For this review, take the finished solid that the model builds, in its own axes (mm). A direction names the side the tool comes from. Coordinates: 2 decimals unless noted, no trailing zeros. Loops run counter-clockwise (first coordinate to the right, second up) from the corner with the lowest first, then second, coordinate; pieces in that order, holes last. Notation, with made-up numbers: (40, 81.5) - (95, 81.5) arc R31 cw to (95, 110.5) - close; hole circle Ø5 at (51, 43). An arc over 180 degrees is marked (long way). One line per item, written item: value. Start each with the question number.
1. Insertion check: pin 1 (6.5 mm diameter, centred on y = 80, z = 108.5, fed in from +X); pin 2 (10 mm diameter, centred on x = 146, y = 134, fed in from +Z); pin 3 (4 mm diameter, centred on y = 122, z = 141.5, fed in from +X); pin 4 (2.5 mm diameter, centred on y = 58, z = 110, fed in from -X). Each pin has a flat end and moves straight along its axis. Give the tip position at first contact, or say it passes through.
2. Take a section at D-D, the plane x = 80.5. State the section outline as (y, z) points.
3. Take a section at C-C, the plane z = 69.5. State the section outline as (x, y) points, and give its area (3 significant figures).
4. Take a section at A-A, the plane x = 139. State the section outline as (y, z) points, and give its area (3 significant figures).
5. The part is to be moulded in two halves that separate along Z. For faces 1 (the face through (59.972, 143.384, 82.338)), 2 (the face through (54, 99, 225)), 3 (the face through (62, 122.3, 83.7)), say which applies: released by +Z, released by -Z, zero draft, split by the parting line, or undercut.
6. Take a section at B-B, the plane x = 104.5. State the section outline as (y, z) points.
7. For faces 4 (the face through (83, 142, 37)), 5 (the face through (59.972, 109.884, 97.338)), 6 (the face through (62, 59.3, 108.7)), 7 (the face through (142, 99.75, 37)), 8 (the face through (83, 57, 37)), list the 3-axis set-ups (+Z, -Z, +X, -X, +Y, -Y) from which the entire face can be reached by the end or side of a thin tool; tool diameter is ignored.
8. To check wall thickness, follow line 1 (Y direction, x = 104.5, z = 42); line 2 (Y direction, x = 53.5, z = 110); line 3 (Z direction, x = 57, y = 121). State the ranges of each line that lie inside material, in increasing order. Write a range as from..to.
```python
from build123d import *

# Parameters (mm, degrees)
F3_DEPTH = 230
F2_W     = 108
F2_H     = 30
F2_W_2   = 100
F2_H_2   = 180
F4_DEPTH = 310
F6_START = 35
F5_R     = 1.5
F6_DEPTH = 36
F7_START = 58
F5_R_2   = 3
F7_DEPTH = 4
F8_START = -44
F2_R     = 2.5
F8_DEPTH = 98


with BuildPart() as f3:
    # F1 (on Top) → F3 (new body)
    with BuildSketch(Plane.XY):
        with BuildLine():
            Line((83, 150), (50, 150))
            Line((50, 150), (50, 50))
            Line((50, 50), (83, 50))
            Line((83, 50), (83, 65))
            Line((83, 65), (158, 65))
            Line((158, 65), (158, 99.75))
            Line((158, 99.75), (126, 99.75))
            Line((126, 99.75), (125.9985464625, 99.75))
            ThreePointArc((125.9985464625, 99.75), (83, 100), (125.9985464625, 100.25))
            Line((125.9985464625, 100.25), (126, 100.25))
            Line((126, 100.25), (158, 100.25))
            Line((158, 100.25), (158, 135))
            Line((158, 135), (83, 135))
            Line((83, 135), (83, 150))
        make_face()
    extrude(amount=F3_DEPTH)

    # F2 (on Front) → F4 (cut)
    with BuildSketch(Plane.XZ):
        with Locations((104, 15)):
            Rectangle(F2_W, F2_H)
        with Locations((108, 135)):
            Rectangle(F2_W_2, F2_H_2)
        Polygon((50, 295), (50, 225), (58, 225), (158, 225), (158, 295), align=None)
    extrude(amount=-F4_DEPTH, mode=Mode.SUBTRACT)

    # F5 (on Right) → F6 (cut)
    with BuildSketch(Plane.YZ.offset(F6_START)):
        with Locations((142, 85)):
            Circle(F5_R)
        with Locations((142, 110)):
            Circle(F5_R)
        with Locations((121, 110)):
            Circle(F5_R)
        with Locations((108.5, 100)):
            Circle(F5_R)
        with Locations((121, 85)):
            Circle(F5_R)
        with Locations((90, 100)):
            Circle(F5_R)
        with Locations((79, 85)):
            Circle(F5_R)
        with Locations((58, 110)):
            Circle(F5_R)
        with Locations((79, 110)):
            Circle(F5_R)
        with Locations((58, 85)):
            Circle(F5_R)
    extrude(amount=F6_DEPTH, mode=Mode.SUBTRACT)

    # F5 (on Right) → F7 (join)
    with BuildSketch(Plane.YZ.offset(F7_START)):
        with Locations((58, 110)):
            Circle(F5_R_2)
        with Locations((58, 110)):
            Circle(F5_R, mode=Mode.SUBTRACT)
        with Locations((79, 110)):
            Circle(F5_R_2)
        with Locations((79, 110)):
            Circle(F5_R, mode=Mode.SUBTRACT)
        with Locations((90, 100)):
            Circle(F5_R_2)
        with Locations((90, 100)):
            Circle(F5_R, mode=Mode.SUBTRACT)
        with Locations((108.5, 100)):
            Circle(F5_R_2)
        with Locations((108.5, 100)):
            Circle(F5_R, mode=Mode.SUBTRACT)
        with Locations((121, 110)):
            Circle(F5_R_2)
        with Locations((121, 110)):
            Circle(F5_R, mode=Mode.SUBTRACT)
        with Locations((142, 110)):
            Circle(F5_R_2)
        with Locations((142, 110)):
            Circle(F5_R, mode=Mode.SUBTRACT)
        with Locations((121, 85)):
            Circle(F5_R_2)
        with Locations((121, 85)):
            Circle(F5_R, mode=Mode.SUBTRACT)
        with Locations((142, 85)):
            Circle(F5_R_2)
        with Locations((142, 85)):
            Circle(F5_R, mode=Mode.SUBTRACT)
        with Locations((79, 85)):
            Circle(F5_R_2)
        with Locations((79, 85)):
            Circle(F5_R, mode=Mode.SUBTRACT)
        with Locations((58, 85)):
            Circle(F5_R_2)
        with Locations((58, 85)):
            Circle(F5_R, mode=Mode.SUBTRACT)
    extrude(amount=F7_DEPTH)

    # F2 (on Front) → F8 (cut)
    with BuildSketch(Plane.XZ.offset(F8_START)):
        with Locations((148.5, 37.5)):
            Circle(F2_R)
    extrude(amount=-F8_DEPTH, mode=Mode.SUBTRACT)


solid = f3.part
```
Solutions:
1. pin 1: x = 62
1. pin 2: z = 45
1. pin 3: x = 58
1. pin 4: through
2. outline: (50, 30) - (150, 30) - (150, 45) - (50, 45) - close
3. outline: (50, 50) - (58, 50) - (58, 150) - (50, 150) - close
3. area: 800 mm2
4. outline: (65, 30) - (99.75, 30) - (99.75, 45) - (65, 45) - close; (100.25, 30) - (135, 30) - (135, 45) - (100.25, 45) - close
4. area: 1,040 mm2
5. face 1: undercut
5. face 2: released by +Z
5. face 3: zero draft
6. outline: (65, 30) - (78.5, 30) - (78.5, 45) - (65, 45) - close; (121.5, 30) - (135, 30) - (135, 45) - (121.5, 45) - close
7. face 4: +Z, -Z, +X, +Y
7. face 5: +X
7. face 6: +Z, +X, +Y, -Y
7. face 7: +Z, -Z, +X
7. face 8: +Z, -Z, +X, -Y
8. line 1: 65..78.5, 121.5..135
8. line 2: 50..56.5, 59.5..77.5, 80.5..119.5, 122.5..140.5, 143.5..150
8. line 3: 30..83.5, 86.5..108.5, 111.5..225
